from build123d import *

# Parameters (mm, degrees)
F0_W     = 320
F0_H     = 50
F1_DEPTH = 2.5
F3_DEPTH = 50
F5_DEPTH = 60
F6_W     = 7.071068
F6_H     = 5
F7_DEPTH = 25
F8_W     = 7.071068
F8_H     = 5
F9_DEPTH = 25


with BuildPart() as f1:
    # F0 (on Front) → F1 (new body, symmetric)
    with BuildSketch(Plane.XZ):
        Rectangle(F0_W, F0_H)
    extrude(amount=F1_DEPTH, both=True)

    # F2 (on face) → F3 (cut)
    with BuildSketch(Plane.XY.offset(25)):
        Polygon((155, 2.5), (160, -2.5), (160, 2.5), align=None)
    extrude(amount=-F3_DEPTH, mode=Mode.SUBTRACT)

    # F4 (on face) → F5 (cut)
    with BuildSketch(Plane.XY.offset(25)):
        Polygon((-155, 2.5), (-160, 2.5), (-160, -2.5), align=None)
    extrude(amount=-F5_DEPTH, mode=Mode.SUBTRACT)

    # F6 (on face) → F7 (cut)
    with BuildSketch(Plane(origin=(78.75, 78.75, 0), x_dir=(-0.707107, 0.707107, 0), z_dir=(0.707107, 0.707107, 0))):
        with Locations((-111.369318, -2.5)):
            Rectangle(F6_W, F6_H)
        with Locations((-111.369318, 2.5)):
            Rectangle(F6_W, F6_H)
    extrude(amount=-F7_DEPTH, mode=Mode.SUBTRACT)

    # F8 (on face) → F9 (cut)
    with BuildSketch(Plane(origin=(-78.75, 78.75, 0), x_dir=(-0.707107, -0.707107, 0), z_dir=(-0.707107, 0.707107, 0))):
        with Locations((111.369318, -2.5)):
            Rectangle(F8_W, F8_H)
        with Locations((111.369318, 2.5)):
            Rectangle(F8_W, F8_H)
    extrude(amount=-F9_DEPTH, mode=Mode.SUBTRACT)


solid = f1.part
Geometry: final body of the model. Coordinates: model frame, mm. A direction names the side the tool comes from. Round coordinates to 2 decimals unless told otherwise and drop trailing zeros. Order: outer loops, then holes, each group sorted by start corner. A loop starts at its lowest first (then second) coordinate and runs counter-clockwise, first axis right, second up.
Q1. Mould query, pull axis Z, two halves, no side actions, for faces 1 (the face through (-152.5, 0, 0.1)), 2 (the face through (157.5, 0, -14.9)), 3 (the face through (-2, 0, -25)). Classes: released by +Z, released by -Z, zero draft, split by the parting line, or undercut.
Result sheet:
face 1: undercut
face 2: zero draft
face 3: released by -Z
Q2. Pin query (flat end, axial travel): pin 1 (2 mm diameter, centred on y = 1, z = -18.5, fed in from +X). Return the tip coordinate at first contact, or that it passes through.
Result sheet:
pin 1: stops at x = 157.5
Q3. Section A-A, the plane y = 1.65. Output: boundary loops of the cut face in (x, z), and give its area (3 significant figures).
Result sheet:
outline: (-155.85, -25) - (155.85, -25) - (155.85, -5) - (154.15, -5) - (154.15, 5) - (155.85, 5) - (155.85, 25) - (-155.85, 25) - (-155.85, 5) - (-154.15, 5) - (-154.15, -5) - (-155.85, -5) - close
area: 15,600 mm2
Q4. Material intervals for probe 1 along X at (y, z) = (2.05, 14); probe 2 along X at (y, z) = (-0.35, -21), sorted ascending.
Result sheet:
probe 1: x = -155.45 to 155.45
probe 2: x = -157.85 to 157.85
Q5. Section B-B, the plane z = -13.5. Output: boundary loops of the cut face in (x, y), and give its area (4 significant figures).
Result sheet:
outline: (-160, -2.5) - (160, -2.5) - (155, 2.5) - (-155, 2.5) - close
area: 1,575 mm2
Q6. Access query for faces 4 (the face through (155, 0, 5)), 5 (the face through (-157.5, 0, 15.1)), 6 (the face through (-155, -1, -5)). Directions: +Z, -Z, +X, -X, +Y, -Y. A direction counts if a zero-diameter tool reaches every point of the face in a straight line with its end or side. Return the directions, or none.
Result sheet:
face 4: +X, -Y
face 5: +Z, -Z, -X, +Y
face 6: -X, -Y
